Could you check a few things on this model? Use its own coordinates, in mm. A direction names the side the tool comes from. Coordinates: 2 decimals unless noted, no trailing zeros. Loops run counter-clockwise (first coordinate to the right, second up) from the corner with the lowest first, then second, coordinate; pieces in that order, holes last. Notation, with made-up numbers: (88.5, 41) - (132.5, 41) arc R19 ccw to (132.5, 51) - close; hole circle Ø1 at (-33, 73.5). An arc over 180 degrees is marked (long way). Use CSV: the item, a comma, the result in double quotes.
from build123d import *

# Parameters (mm, degrees)
SKETCH1_W               = 35
SKETCH1_H               = 70
BOSS_EXTRUDE1_DEPTH     = 10
BOSS_EXTRUDE3_DEPTH     = 310
BOSS_EXTRUDE4_DEPTH     = 240
SKETCH6_R               = 2
CUT_EXTRUDE1_DEPTH      = 280
LPATTERN1_COUNT         = 2
LPATTERN1_PITCH         = 100
LPATTERN1_COL_COUNT     = 2
LPATTERN1_COL_PITCH     = 100
CUT_EXTRUDE2_DEPTH      = 295
CUT_EXTRUDE2_DEPTH_BACK = 10
SKETCH10_W              = 83
SKETCH10_H              = 70
SKETCH11_W              = 164
SKETCH11_H              = 5
BOSS_EXTRUDE5_DEPTH     = 86


with BuildPart() as part:
    # Sketch1 → Boss-Extrude1 (new body)
    with BuildSketch(Plane(origin=(0, 0, 0), x_dir=(1, 0, 0), z_dir=(0, 1, 0))):
        Polygon((-100, 150), (-150, 85), (-150, -85), (-100, -150), (100, -150), (150, -85), (150, 85), (100, 150), align=None)
        with Locations((-122.5, 0)):
            Rectangle(SKETCH1_W, SKETCH1_H, mode=Mode.SUBTRACT)
        with Locations((122.5, 0)):
            Rectangle(SKETCH1_W, SKETCH1_H, mode=Mode.SUBTRACT)
    extrude(amount=BOSS_EXTRUDE1_DEPTH)

    # Sketch4 → Boss-Extrude3 (add)
    with BuildSketch(Plane(origin=(0, 10, 0), x_dir=(1, 0, 0), z_dir=(0, 1, 0))):
        Polygon((-12.5, -73), (12.5, -73), (12.5, -68), (7.5, -68), (7.5, -58), (12.5, -58), (12.5, -53), (-12.5, -53), (-12.5, -58), (-7.5, -58), (-7.5, -68), (-12.5, -68), align=None)
        Polygon((-150, 85), (-150, -85), (-145, -85), (-145, -80), (-135, -80), (-135, -85), (-130, -85), (-130, -65), (-145, -65), (-145, 65), (-130, 65), (-130, 85), (-135, 85), (-135, 80), (-145, 80), (-145, 85), align=None)
        Polygon((145, 85), (150, 85), (150, -85), (145, -85), (145, -80), (135, -80), (135, -85), (130, -85), (130, -65), (145, -65), (145, 65), (130, 65), (130, 85), (135, 85), (135, 80), (145, 80), align=None)
    boss_extrude3 = extrude(amount=BOSS_EXTRUDE3_DEPTH)

    # Sketch5 → Boss-Extrude4 (add)
    with BuildSketch(Plane(origin=(0, 10, 0), x_dir=(1, 0, 0), z_dir=(0, 1, 0))):
        Polygon((-145, -47), (-85, -47), (-85, -40), (85, -40), (85, -47), (145, -47), (145, -50), (82, -50), (82, -43), (-82, -43), (-82, -50), (-145, -50), align=None)
    boss_extrude4 = extrude(amount=BOSS_EXTRUDE4_DEPTH)

    # Sketch6 → Cut-Extrude1 (cut)
    with BuildSketch(Plane(origin=(0, 10, 0), x_dir=(1, 0, 0), z_dir=(0, 1, 0))):
        with Locations(Location((-65, -80, 0), (0, 0, 270))):
            Circle(SKETCH6_R)
        with Locations(Location((-65, -108, 0), (0, 0, 270))):
            Circle(SKETCH6_R)
        with Locations(Location((65, -108, 0), (0, 0, 90))):
            Circle(SKETCH6_R)
        with Locations(Location((65, -80, 0), (0, 0, 90))):
            Circle(SKETCH6_R)
    cut_extrude1 = extrude(amount=-CUT_EXTRUDE1_DEPTH, mode=Mode.SUBTRACT)

    # Mirror1: Boss-Extrude3, Boss-Extrude4, Cut-Extrude1 across plane
    add(boss_extrude3.mirror(Plane.XY))
    add(boss_extrude4.mirror(Plane.XY))
    add(cut_extrude1.mirror(Plane.XY), mode=Mode.SUBTRACT)

    # Sketch9 → Revolve1 (revolve)
    with BuildSketch(Plane(origin=(0, 0, 0), x_dir=(0, 0, -1), z_dir=(1, 0, 0))):
        with BuildLine():
            Line((117.5, 0), (117.5, -4))
            ThreePointArc((117.5, -4), (120.328427125, -2.828427125), (121.5, 0))
            Line((121.5, 0), (117.5, 0))
        make_face()
    revolve1 = revolve(axis=Axis((0, 0, -117.5), (0, -1, 0)))

    # LPattern1: Revolve1 ×2
    with Locations(*[(-i * LPATTERN1_PITCH, 0, 0) for i in range(1, LPATTERN1_COUNT)]):
        add(revolve1)

    # LPattern1 col: Revolve1 ×2
    with Locations(*[(i * LPATTERN1_COL_PITCH, 0, 0) for i in range(1, LPATTERN1_COL_COUNT)]):
        add(revolve1)

    # Mirror2: Revolve1 across plane
    add(revolve1.mirror(Plane.XY))

    # Mirror2 copy 1 sketch → Mirror2 copy 1 (revolve)
    with BuildSketch(Plane(origin=(-100, 0, 0), x_dir=(0, 0, 1), z_dir=(1, 0, 0))):
        with BuildLine():
            Line((117.5, 0), (117.5, 4))
            ThreePointArc((117.5, 4), (120.328427125, 2.828427125), (121.5, 0))
            Line((121.5, 0), (117.5, 0))
        make_face()
    revolve(axis=Axis((-100, 0, 117.5), (0, 1, 0)))

    # Mirror2 copy 2 sketch → Mirror2 copy 2 (revolve)
    with BuildSketch(Plane(origin=(100, 0, 0), x_dir=(0, 0, 1), z_dir=(1, 0, 0))):
        with BuildLine():
            Line((117.5, 0), (117.5, 4))
            ThreePointArc((117.5, 4), (120.328427125, 2.828427125), (121.5, 0))
            Line((121.5, 0), (117.5, 0))
        make_face()
    revolve(axis=Axis((100, 0, 117.5), (0, 1, 0)))

    # Sketch10 → Cut-Extrude2 (cut, two sides: drawn at the far end of the back side and taken through both)
    with BuildSketch(Plane(origin=(-145, 0, 0), x_dir=(0, 0, -1), z_dir=(1, 0, 0)).offset(-CUT_EXTRUDE2_DEPTH_BACK)):
        with Locations((1.5, 285)):
            Rectangle(SKETCH10_W, SKETCH10_H)
    extrude(amount=CUT_EXTRUDE2_DEPTH + CUT_EXTRUDE2_DEPTH_BACK, mode=Mode.SUBTRACT)

    # Sketch11 → Boss-Extrude5 (add)
    with BuildSketch(Plane.XY.offset(43)):
        with Locations((0, 137.5)):
            Rectangle(SKETCH11_W, SKETCH11_H)
    extrude(amount=-BOSS_EXTRUDE5_DEPTH)


solid = part.part
(1) Will these pins go through, and if not, where does the flat tip stop? pin 1 (10 mm diameter, centred on x = -38, y = 51, fed in from -Z); pin 2 (6 mm diameter, centred on x = -67.5, y = 163, fed in from +Z); pin 3 (4 mm diameter, centred on x = 9, y = 113.5, fed in from -Z); pin 4 (3.5 mm diameter, centred on x = -65, z = 108, fed in from +Y).
Computed:
pin 1,"stops at z = -43"
pin 2,"stops at z = 43"
pin 3,"stops at z = -73"
pin 4,"passes through"
(2) Suppose I cut it at A-A (x = 17.5). Write out the boundary of the cut face in (y, z).
Computed:
outline,"(0, -150) - (10, -150) - (10, -43) - (250, -43) - (250, -40) - (140, -40) - (140, 40) - (250, 40) - (250, 43) - (10, 43) - (10, 150) - (0, 150) - close; hole (10, -40) - (135, -40) - (135, 40) - (10, 40) - close"
(3) Which directions (+Z, -Z, +X, -X, +Y, -Y) give clear straight access to the entire face, cutting with the end or side of a thin tool? Please do faces 4 (the face through (-2, 10, -1)), 5 (the face through (0, 163, 73)), 6 (the face through (140, 5, 0)), 7 (the face through (-130, 163, -75)).
Computed:
face 4,"none"
face 5,"+Z, +Y"
face 6,"+Y, -Y"
face 7,"-Z, +Y"
(4) Thinking about a two-plate mould opening in X: for faces 1 (the face through (150, 158, 1)), 2 (the face through (-113, 128, 50)), 3 (the face through (142, 320, -69)), which applies, +X half, -X half, draft (parallel to the pull), parting line (faces both ways), or undercut?
Computed:
face 1,"+X half"
face 2,"undercut"
face 3,"draft"
(5) Please list where these lines run through material, in increasing order: line 1 (X direction, y = 188.5, z = 41.5); line 2 (Z direction, x = 65, y = 2); line 3 (X direction, y = 294, z = 57).
Computed:
line 1,"x = -150 to -145, -85 to 85, 145 to 150"
line 2,"z = -150 to -110, -106 to -82, -78 to 78, 82 to 106, 110 to 150"
line 3,"x = -150 to -145, -12.5 to 12.5, 145 to 150"
(6) Suppose I cut it at C-C (x = -91). Write out the boundary of the cut face in (y, z), plus the area to 3 significant figures.
Computed:
outline,"(0, -150) - (10, -150) - (10, -50) - (250, -50) - (250, -47) - (10, -47) - (10, 47) - (250, 47) - (250, 50) - (10, 50) - (10, 150) - (0, 150) - close"
area,"4,440 mm²"
(7) Suppose I cut it at B-B (y = 216). State how many separate pieces and enclosed holes the cut face has, plus the area to 3 significant figures.
Computed:
separate pieces,"3"
enclosed holes,"1"
area,"5,320 mm²"
